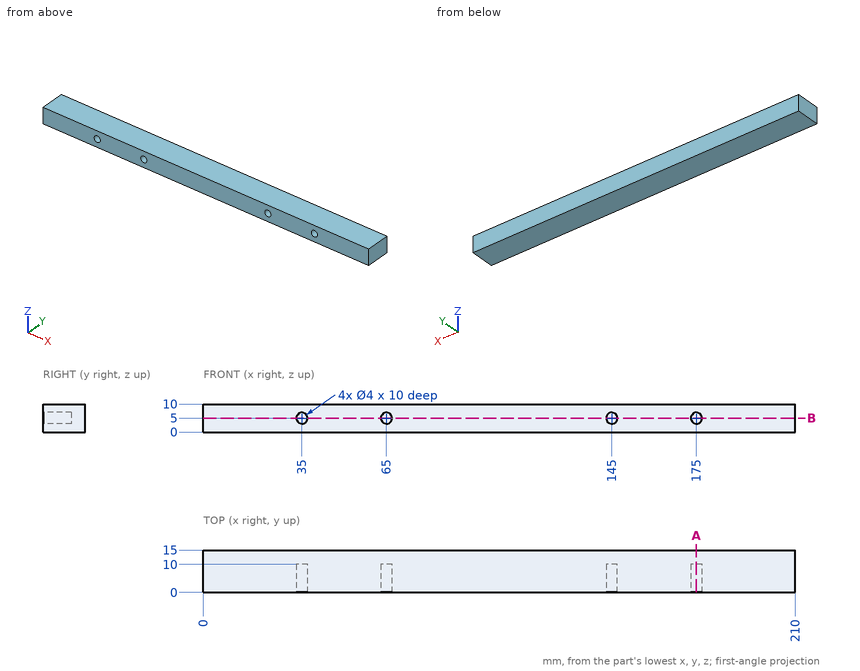
Print and shaded views of the part. All mm, measured from the part's lowest x, y and z. Round coordinates to 2 decimals unless told otherwise and drop trailing zeros. Write each loop counter-clockwise with the first axis right and the second up, starting at its lowest first coordinate (ties: lowest second). Pieces come first, ordered by that corner, then holes. Notation, with made-up numbers: (82.5, 69) - (139.5, 69) arc R16 cw to (139.5, 90) - close; hole circle Ø10 at (41.5, -15). An arc over 180 degrees is marked (long way). Write each question's results on one line, items separated by ' | '. Start each with the question number.
Item 1: Saw through at B-B (z = 5). Write the cut outline in (x, y).
Item 2: Wall check: L1, parallel to Z at x = 145, y = 3.75. Give the ranges that are in metal, low to high. Write a range as [from, to].
Item 3: Saw through at A-A (x = 175). Write the cut outline in (y, z), and give its area (3 significant figures).
Item 4: Drop a flat-ended pin along its axis: P1, Ø2.5, axis at x = 35, z = 5, coming from the -Y side. Give the stop position or say it passes through.
Results are:
1) outline: (0, 0) - (33, 0) - (33, 10) - (37, 10) - (37, 0) - (63, 0) - (63, 10) - (67, 10) - (67, 0) - (143, 0) - (143, 10) - (147, 10) - (147, 0) - (173, 0) - (173, 10) - (177, 10) - (177, 0) - (210, 0) - (210, 15) - (0, 15) - close
2) L1: z = [0, 3], [7, 10]
3) outline: (0, 0) - (15, 0) - (15, 10) - (0, 10) - (0, 7) - (10, 7) - (10, 3) - (0, 3) - close | area: 110 mm²
4) P1: stops at y = 10
